Work out the finished part from the listing and answer in its coordinate system (mm). A direction names the side the tool comes from. Round coordinates to 2 decimals unless told otherwise and drop trailing zeros. Loops run counter-clockwise (first coordinate to the right, second up) from the corner with the lowest first, then second, coordinate; pieces in that order, holes last.
```python
from build123d import *

# Parameters (mm, degrees)
SKETCH1_R           = 16.5
BOSS_EXTRUDE1_DEPTH = 23
SKETCH2_R           = 18.5
BOSS_EXTRUDE2_DEPTH = 23
SKETCH3_R           = 6
BOSS_EXTRUDE3_DEPTH = 6
BOSS_EXTRUDE4_DEPTH = 12
CIRPATTERN1_COUNT   = 6
SKETCH8_R           = 15.5
BOSS_EXTRUDE5_DEPTH = 2
SKETCH10_W          = 6
SKETCH10_H          = 13.585847052
BOSS_EXTRUDE6_DEPTH = 5.02500011


with BuildPart() as part:
    # Sketch1 → Boss-Extrude1 (new body)
    with BuildSketch(Plane.XY):
        Circle(SKETCH1_R)
    extrude(amount=-BOSS_EXTRUDE1_DEPTH)

    # Sketch2 → Boss-Extrude2 (add)
    with BuildSketch(Plane(origin=(0, 0, -23), x_dir=(-1, 0, 0), z_dir=(0, 0, -1))):
        Circle(SKETCH2_R)
    extrude(amount=BOSS_EXTRUDE2_DEPTH)

    # Sketch3 → Boss-Extrude3 (add)
    with BuildSketch(Plane(origin=(0, 0, -46), x_dir=(-1, 0, 0), z_dir=(0, 0, -1))):
        with Locations((0, 7)):
            Circle(SKETCH3_R)
    extrude(amount=BOSS_EXTRUDE3_DEPTH)

    # Sketch4 → Boss-Extrude4 (add)
    with BuildSketch(Plane(origin=(0, 0, -52), x_dir=(-1, 0, 0), z_dir=(0, 0, -1))):
        with BuildLine():
            Line((-1.658312395, 9.5), (1.658312395, 9.5))
            ThreePointArc((1.658312395, 9.5), (0, 4), (-1.658312395, 9.5))
        make_face()
    extrude(amount=BOSS_EXTRUDE4_DEPTH)

    # Sketch7 → M3x0.5 Tapped Hole1 (revolve, cut)
    with BuildSketch(Plane(origin=(-15.5, 0, -46), x_dir=(0, 1, 0), z_dir=(1, 0, 0))):
        Polygon((0, 0), (0, 10.751081174), (1.25, 10.0000054), (1.25, 0.275), (1.525, 0), align=None)
    m3x0_5_tapped_hole1 = revolve(axis=Axis((-15.5, 0, -52.35), (0, 0, 1)), mode=Mode.SUBTRACT)

    # CirPattern1: M3x0.5 Tapped Hole1 ×6 about axis
    cirpattern1_axis = Axis((0, 0, 0), (0, 0, 1))
    for i in range(1, CIRPATTERN1_COUNT):
        add(m3x0_5_tapped_hole1.rotate(cirpattern1_axis, i * 360 / CIRPATTERN1_COUNT), mode=Mode.SUBTRACT)

    # Sketch8 → Boss-Extrude5 (add)
    with BuildSketch(Plane.XY):
        Circle(SKETCH8_R)
    extrude(amount=BOSS_EXTRUDE5_DEPTH)

    # Sketch10 → Boss-Extrude6 (add)
    with BuildSketch(Plane.XY.offset(2)):
        with Locations((-15.5, 0)):
            Rectangle(SKETCH10_W, SKETCH10_H)
    extrude(amount=BOSS_EXTRUDE6_DEPTH)


solid = part.part
```
1. Determine the mould class of faces 4 (the face through (8.97, 13.15, -40.93)), 5 (the face through (-16, 0, 7.025)), 6 (the face through (0.78, 12.95, -48.96)) for opening direction X: +X half, -X half, draft (parallel to the pull), parting line (faces both ways), or undercut.
Answer key:
face 4: undercut
face 5: draft
face 6: parting line
2. Given pin 1 (1.7 mm diameter, centred on x = -0.5, z = -58.5, fed in from +Y); pin 2 (1.5 mm diameter, centred on y = -9, z = -46, fed in from +X); pin 3 (1.5 mm diameter, centred on x = 7.75, y = -13.42, fed in from -Z), each flat-ended and moving along its own axis, determine where each tip first touches the part or whether it passes through.
Answer key:
pin 1: stops at y = 9.5
pin 2: stops at x = 16.56
pin 3: stops at z = -35.7
3. Consider probe 1 along Y at (x, z) = (-7, -40); probe 2 along Z at (x, y) = (-16, 3) (3 decimals); probe 3 along Z at (x, y) = (13, 1). Determine where each line is inside the solid, lowest interval first.
Answer key:
probe 1: y = -17.12 to -14.42, -12.42 to 12.42, 14.42 to 17.12
probe 2: z = -46 to 0, 2 to 7.025
probe 3: z = -46 to 2
4. Which of the six approach directions +Z, -Z, +X, -X, +Y, -Y give full straight-line access (tool end or side, diameter ignored) to faces 1 (the face through (8.23, -12.27, -40.93)), 2 (the face through (-16, -6.793, 4)), 3 (the face through (5, 15, 0))?
Answer key:
face 1: -Z
face 2: +Z, +X, -X, -Y
face 3: none
5. Find section C-C (y = -4.5). Write down the section's boundary in (x, z) (1 decimal), then the cut area to 3 significant figures.
Answer key:
outline: (-18.5, 2) - (-14.8, 2) - (-14.8, 0) - (-15.9, 0) - (-15.9, -23) - (-17.9, -23) - (-17.9, -46) - (17.9, -46) - (17.9, -23) - (15.9, -23) - (15.9, 0) - (14.8, 0) - (14.8, 2) - (-12.5, 2) - (-12.5, 7) - (-18.5, 7) - close
area: 1,650 mm2
6. Find section A-A (x = 0). Write down the section's boundary in (y, z), then the cut area to 3 significant figures.
Answer key:
outline: (-18.5, -46) - (1, -46) - (1, -52) - (4, -52) - (4, -64) - (9.5, -64) - (9.5, -52) - (13, -52) - (13, -46) - (18.5, -46) - (18.5, -23) - (16.5, -23) - (16.5, 0) - (15.5, 0) - (15.5, 2) - (-15.5, 2) - (-15.5, 0) - (-16.5, 0) - (-16.5, -23) - (-18.5, -23) - close
area: 1,810 mm2
7. Find section D-D (x = 12). Write down the section's boundary in (y, z), then the cut area to 3 significant figures.
Answer key:
outline: (-14.08, -46) - (14.08, -46) - (14.08, -23) - (11.32, -23) - (11.32, 0) - (9.81, 0) - (9.81, 2) - (-9.81, 2) - (-9.81, 0) - (-11.32, 0) - (-11.32, -23) - (-14.08, -23) - close
area: 1,210 mm2
8. Find section B-B (z = -45). Write down the section's boundary in (x, y).
Answer key:
outline: circle Ø37 at (0, 0); hole circle Ø2.5 at (-15.5, 0); hole circle Ø2.5 at (-7.75, -13.42); hole circle Ø2.5 at (-7.75, 13.42); hole circle Ø2.5 at (7.75, -13.42); hole circle Ø2.5 at (7.75, 13.42); hole circle Ø2.5 at (15.5, 0)
